Read the model definition and answer for the solid it produces. Units are mm, in the model's axes. Give positions to 0.01 mm unless a question says otherwise; leave off trailing zeros. Return JSON: item names as keys, results as strings. Group by question number.
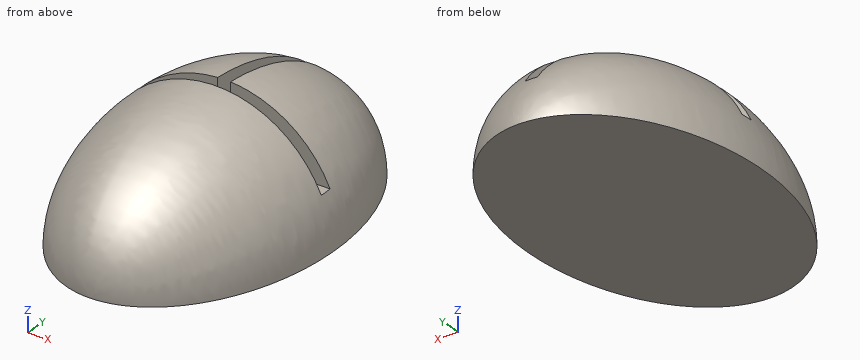
```python
from build123d import *

# Parameters (mm, degrees)
F3_DEPTH      = 25
F3_DEPTH_BACK = 25
F5_START      = 1.48
F5_DEPTH      = 10.02


with BuildPart() as f1:
    # F0 (on Top) → F1 (revolve)
    with BuildSketch(Plane.XY):
        with BuildLine():
            Line((0, 1.8567474326), (0, 5.25))
            add(Edge.make_bspline(
                [(0, 5.25), (-3.5, 5.25), (-3.5, 0), (-3.5, -5.25), (0, -5.25)],
                knots=[0, 0, 0, 1.5707963268, 1.5707963268, 3.1415926536, 3.1415926536, 3.1415926536], degree=2, weights=[1, 0.7071067812, 1, 0.7071067812, 1]))
            Line((0, -5.25), (0, 0))
            Line((0, 0), (0, 1.8567474326))
        make_face()
    revolve(axis=Axis((0, 3.5533737163, 0), (0, 1, 0)))

    # F2 (on Right) → F3 (cut, two sides)
    with BuildSketch(Plane.YZ) as f3_sk:
        Polygon((6.3744364306, 0), (0, 0), (-6.297763437, 0), (-6.297763437, -3.5955796484), (6.3744364306, -3.5955796484), align=None)
    extrude(amount=-F3_DEPTH, mode=Mode.SUBTRACT)
    extrude(f3_sk.sketch, amount=F3_DEPTH_BACK, mode=Mode.SUBTRACT)

    # F4 (on Top) → F5 (cut)
    with BuildSketch(Plane.XY.offset(F5_START)):
        Polygon((-4.4482909143, 0), (0, 0), (4.5133754611, 0), (4.5133754611, 0.38), (0.1900000061, 0.38), (0.1900000061, 5.200644955), (0.1900000061, 5.4544974118), (-0.19, 5.4544974118), (-0.19, 5.200644955), (-0.19, 0.38), (-4.4482909143, 0.38), align=None)
    extrude(amount=F5_DEPTH, mode=Mode.SUBTRACT)


solid = f1.part
```
1. Flat-ended cylindrical pins translate along their axes: P1, Ø1.5, axis at x = 0, y = 1, coming from the +Z side; P2, Ø2, axis at x = -1, z = 2.5, coming from the +Y side; P3, Ø1, axis at x = -1.5, z = 2.5, coming from the -Y side. Find the tip coordinate at first contact, or state that the pin passes through.
2. Straight lines are drawn through the part: line 1 along Y through (x, z) = (-0.75, 2.05); line 2 along Z through (x, y) = (0, 3); line 3 along Y through (x, z) = (1.5, 2.6). For each, find the intervals that lie inside material, in ascending order.
3. Find section A-A (z = 2.35). State how many separate pieces and enclosed holes the cut face has, and give its area (3 significant figures).
Result:
{
 "1": {"P1": "stops at z = 3.49", "P2": "stops at y = 4.6", "P3": "stops at y = -3.8"},
 "2": {"line 1": "y = -4.1 to 0, 0.38 to 4.1", "line 2": "z = 0 to 1.48", "line 3": "y = -2.7 to 0, 0.38 to 2.7"},
 "3": {"separate pieces": "3", "enclosed holes": "0", "area": "28.4 mm2"}
}
